Read the model definition and answer for the solid it produces. Units are mm, in the model's axes. Give positions to 0.01 mm unless a question says otherwise; leave off trailing zeros. Loops run counter-clockwise (first coordinate to the right, second up) from the corner with the lowest first, then second, coordinate; pieces in that order, holes last. Notation, with made-up numbers: (87.5, 59) - (122.5, 59) arc R7 cw to (122.5, 63) - close; hole circle Ø10 at (83.25, -38.75). An arc over 180 degrees is marked (long way). Write item = value, one per line.
Autodesk Inventor part; units mm, degrees
ref_plane "YZ Plane" through (0, 0, 0) normal (1, 0, 0) x (0, 1, 0)
ref_plane "XZ Plane" through (0, 0, 0) normal (0, 1, 0) x (-1, 0, 0)
ref_plane "XY Plane" through (0, 0, 0) normal (0, 0, 1) x (1, 0, 0)
sketch "Sketch1" plane through (0, 0, 0) normal (0, 0, 1) x (1, 0, 0)
  line L0 (-31.75, 5.08) -> (31.75, 5.08)
  line L1 (31.75, 5.08) -> (31.75, -5.08)
  line L2 (31.75, -5.08) -> (-31.75, -5.08)
  line L3 (-31.75, -5.08) -> (-31.75, 5.08)
  point P0 (0, 0)
  dimension "d0" = 63.5
  dimension "d3" = 31.75
  dimension "d4" = 10.16
  dimension "d17" = 5.08
extrude "Extrusion1" add sketch "Sketch1" along normal blind 76.2
sketch "Sketch3" plane through (0, 0, 76.2) normal (0, 0, 1) x (1, 0, 0)
  line L0 (-27.25, 0.3875) -> (27.25, 0.3875)
  line L1 (27.25, 0.3875) -> (27.25, -0.3745)
  line L2 (27.25, -0.3745) -> (-27.25, -0.3745)
  line L3 (-27.25, -0.3745) -> (-27.25, 0.3875)
  line L4 (-31.75, 5.08) -> (-31.75, -5.08)
  point P0 (0, 0)
  point P1 (-27.25, 0.0065)
  dimension "d6" = 0.762
  dimension "d7" = 54.5
  dimension "d8" = 4.5
extrude "Extrusion2" cut sketch "Sketch3" against normal blind 85.1
sketch "Sketch8" plane through (0, 0, 76.2) normal (0, 0, 1) x (1, 0, 0)
  line L0 (-31.75, 5.08) -> (-31.75, -5.08)
  line L1 (31.75, -5.08) -> (31.75, 5.08)
  line L2 (-31.75, -5.08) -> (31.75, -5.08)
  line L3 (31.75, -5.08) -> (31.75, 0.3875)
  line L4 (31.75, 0.3875) -> (-31.75, 0.3875)
  line L5 (-31.75, 0.3875) -> (-31.75, -5.08)
  line L6 (-27.25, 0.3875) -> (27.25, 0.3875)
  point P0 (0, 0)
  point P1 (-31.75, 0.3875)
  dimension "d30" = 0
extrude "Extrusion6" cut sketch "Sketch8" against normal blind 76.2
sketch "Sketch9" plane through (-31.75, 5.08, 0) normal (0, 1, 0) x (1, 0, 0)
  line L0 (63.5, 0) -> (0, 0)
  line L1 (0, 0) -> (0, -76.2)
  line L2 (63.5, -76.2) -> (0, -76.2)
  line L3 (63.5, 0) -> (63.5, -76.2)
  line L4 (12.7, -12.7) -> (50.8, -12.7)
  line L5 (50.8, -12.7) -> (50.8, -63.5)
  line L6 (50.8, -63.5) -> (12.7, -63.5)
  line L7 (12.7, -63.5) -> (12.7, -12.7)
  point P0 (31.75, 0)
  dimension "d33" = 12.7
extrude "Extrusion7" cut sketch "Sketch9" against normal blind 25.4 contours L4 L5 L6 L7
sketch "Sketch11" plane through (-31.75, 5.08, 0) normal (0, 1, 0) x (1, 0, 0)
  circle A0 centre (61.25, -72.39) radius 1.05
  line L0 (59, -76.2) -> (63.5, -76.2)
  line L1 (59, 0) -> (59, -76.2)
  circle A1 centre (2.25, -72.39) radius 1.05
  line L2 (0, 0) -> (0, -76.2)
  line L3 (0, -76.2) -> (4.5, -76.2)
  circle A2 centre (2.25, -3.81) radius 1.05
  circle A3 centre (61.25, -3.81) radius 1.05
  line L4 (4.5, 0) -> (0, 0)
  line L5 (63.5, 0) -> (59, 0)
  line L6 (50.8, -12.7) -> (50.8, -63.5)
  line L7 (50.8, -63.5) -> (12.7, -63.5)
  line L8 (12.7, -63.5) -> (12.7, -12.7)
  line L9 (12.7, -12.7) -> (50.8, -12.7)
  line L10 (63.5, 0) -> (0, 0)
  line L11 (0, 0) -> (0, -76.2)
  line L12 (63.5, -76.2) -> (0, -76.2)
  line L13 (63.5, 0) -> (63.5, -76.2)
  point P0 (31.75, -76.2)
  dimension "d37" = 2.1
  dimension "d38" = 3.81
  dimension "d39" = 2.25
  dimension "d40" = 2.25
  dimension "d41" = 2.1
  dimension "d42" = 3.81
  dimension "d43" = 2.1
  dimension "d44" = 2.1
  dimension "d45" = 3.81
  dimension "d46" = 3.81
  dimension "d47" = 2.25
  dimension "d48" = 2.25
extrude "Extrusion8" cut sketch "Sketch11" against normal blind 25.4 contours A0 | A1 | A2 | A3
fillet "Fillet1" radius 1.905 1 edges at (0, 5.08, 0)
sketch "Sketch13" plane through (-31.75, 5.08, 76.2) normal (0, 1, 0) x (1, 0, 0)
  point P0 (31.75, 76.2)
sketch "Sketch14" plane through (-31.75, 5.08, 76.2) normal (0, 1, 0) x (1, 0, 0)
  line L0 (19.685, 1.905) -> (43.815, 1.905)
  line L1 (43.815, 1.905) -> (43.815, 5.715)
  line L2 (43.815, 5.715) -> (19.685, 5.715)
  line L3 (19.685, 5.715) -> (19.685, 1.905)
  line L4 (63.5, 76.2) -> (0, 76.2)
  line L5 (0, 74.295) -> (0, 0)
  line L6 (63.5, 74.295) -> (63.5, 0)
  line L7 (63.5, 0) -> (0, 0)
  point P0 (31.75, 76.2)
  dimension "d54" = 1.905
  dimension "d55" = 3.81
  dimension "d61" = 24.13
  dimension "d62" = 63.5
  dimension "d63" = 19.685
extrude "Extrusion9" cut sketch "Sketch14" against normal blind 25.4
sketch "Sketch15" plane through (0, 0, 0) normal (0, 0, -1) x (-1, 0, 0)
  line L0 (31.75, 0.3875) -> (-31.75, 0.3875)
  line L1 (-31.75, 0.3875) -> (-31.75, 5.08)
  line L2 (31.75, 0.3875) -> (-31.75, 0.3875)
  line L3 (-31.75, 0.3875) -> (-31.75, 1.0225)
  line L4 (-31.75, 1.0225) -> (31.75, 1.0225)
  line L5 (31.75, 1.0225) -> (31.75, 0.3875)
  point P0 (0, 0)
  dimension "d58" = 0.635
extrude "Extrusion10" cut sketch "Sketch15" against normal blind 76.2
properties part number "Scanner_Test_Bot"
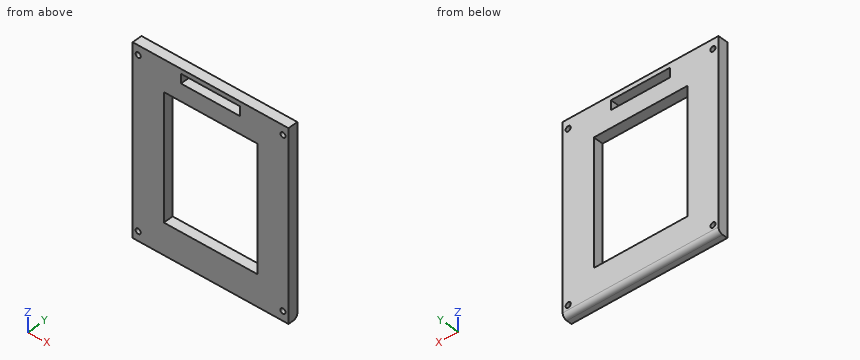
1) A cutting plane is placed at D-D on z = 3.81. Determine the outline of the cut face in (x, y), then the cut area to 3 significant figures.
Output:
outline = (-31.75, 1.02) - (-30.55, 1.02) - (-30.55, 5.08) - (-31.75, 5.08) - close; (-28.45, 1.02) - (28.45, 1.02) - (28.45, 5.08) - (-28.45, 5.08) - close; (30.55, 1.02) - (31.75, 1.02) - (31.75, 5.08) - (30.55, 5.08) - close
area = 241 mm²
2) A cutting plane is placed at C-C on z = 72.39. Give the number of separate pieces and of enclosed holes in the cut face, then the cut area to 3 significant figures.
Output:
separate_pieces = 4
enclosed_holes = 0
area = 143 mm²
3) A cutting plane is placed at A-A on z = 39. Determine the outline of the cut face in (x, y).
Output:
outline = (-31.75, 1.02) - (-19.05, 1.02) - (-19.05, 5.08) - (-31.75, 5.08) - close; (19.05, 1.02) - (31.75, 1.02) - (31.75, 5.08) - (19.05, 5.08) - close
4) This flat-tipped pin is pushed along its axis until it touches: P1, Ø3.5, axis at x = 29.5, z = 3.81, coming from the +Y side. Where does it stop, or does it pass through?
Output:
P1 = 5.08
5) Find the intervals of material crossed by probe 1 along Z at (x, y) = (8, 3.3) (3 decimals); probe 2 along X at (y, z) = (2.65, 3.81); probe 3 along X at (y, z) = (2.1, 72.39) (3 decimals), in increasing order.
Output:
probe_1 = 0.004 to 12.7, 63.5 to 70.485, 74.295 to 76.2
probe_2 = -31.75 to -30.55, -28.45 to 28.45, 30.55 to 31.75
probe_3 = -31.75 to -30.55, -28.45 to -12.065, 12.065 to 28.45, 30.55 to 31.75
6) A cutting plane is placed at B-B on x = -29.5. Determine the outline of the cut face in (y, z) (1 decimal), then the cut area to 3 significant figures.
Output:
outline = (1, 0) - (3.2, 0) arc R1.9 ccw to (5.1, 1.9) - (5.1, 2.8) - (1, 2.8) - close; (1, 4.9) - (5.1, 4.9) - (5.1, 71.3) - (1, 71.3) - close; (1, 73.4) - (5.1, 73.4) - (5.1, 76.2) - (1, 76.2) - close
area = 291 mm²
